The listing builds one solid part. Answer for the finished solid, in the listing's coordinates (mm). A direction names the side the tool comes from. Give positions to 0.01 mm unless a question says otherwise; leave off trailing zeros. Write each loop counter-clockwise with the first axis right and the second up, starting at its lowest first coordinate (ties: lowest second). Pieces come first, ordered by that corner, then holes. Notation, with made-up numbers: (-29.5, 26.5) - (0.5, 26.5) arc R21 cw to (0.5, 57.5) - close; hole circle Ø7 at (81, 60). An arc over 180 degrees is marked (long way). One line per question, with ' | ' between items. Start each with the question number.
1. The mould has two halves that part along X. Classify faces 6 (the face through (0, 0, 0)), 7 (the face through (3.75, 16, 10)), 8 (the face through (-19, 0, 2)), 9 (the face through (20, 0, 12)): +X half, -X half, draft (parallel to the pull), parting line (faces both ways), or undercut.
2. A cutting plane is placed at B-B (z = 16.75). Determine the outline of the cut face in (x, y), then the cut area to 3 significant figures.
3. For faces 1 (the face through (0, -21.5, 10)), 2 (the face through (-3.75, 16, 10)), 3 (the face through (16, 13.9, 11.5)), 4 (the face through (0, 5, 20)), 5 (the face through (-1.19, -16.87, 16.84)), determine the directions among +Z, -Z, +X, -X, +Y, -Y from which every point of the face is accessible in a straight line to the end or side of a thin tool.
4. A cutting plane is placed at C-C (y = 11). Determine the outline of the cut face in (x, z), then the cut area to 3 significant figures.
5. Find the intervals of material crossed by L1, parallel to X at y = 17.5, z = 10; L2, parallel to X at y = 10.75, z = 10; L3, parallel to Z at x = -14, y = 16, in increasing order. Write a range as from..to.
6. Given P1, Ø5.5, axis at x = 0.5, y = -12, coming from the +Z side, flat-ended and moving along its own axis, determine where the tip first touches the part or whether it passes through.
7. A cutting plane is placed at A-A (y = 17.5). Determine the outline of the cut face in (x, z), then the cut area to 3 significant figures.
8. A cutting plane is placed at D-D (z = 11.5). State how many separate pieces and enclosed holes the cut face has, then the cut area to 3 significant figures.
```python
from build123d import *

# Parameters (mm, degrees)
SKETCH1_W                                           = 40
SKETCH1_H                                           = 43
BOSS_EXTRUDE1_DEPTH                                 = 20
SKETCH2_W                                           = 7.5
SKETCH2_H                                           = 20
CUT_EXTRUDE1_DEPTH                                  = 10
M6_TAPPED_HOLE1_D                                   = 5
M6_TAPPED_HOLE1_DEPTH                               = 15
M6_TAPPED_HOLE1_TIP                                 = 1.502151548
FILLET1_R                                           = 5
CHAMFER1_SIZE                                       = 0.5
CBORE_FOR_M6_HEX_SOCKET_HEAD_CAP_SCREW1_D           = 6.4
CBORE_FOR_M6_HEX_SOCKET_HEAD_CAP_SCREW1_CBORE_D     = 11
CBORE_FOR_M6_HEX_SOCKET_HEAD_CAP_SCREW1_CBORE_DEPTH = 6.4
M5_TAPPED_HOLE1_D                                   = 4.2
M5_TAPPED_HOLE1_DEPTH                               = 12.4
M5_TAPPED_HOLE1_TIP                                 = 1.2618073


with BuildPart() as part:
    # Sketch1 → Boss-Extrude1 (new body)
    with BuildSketch(Plane.XY):
        Rectangle(SKETCH1_W, SKETCH1_H)
    extrude(amount=BOSS_EXTRUDE1_DEPTH)

    # Sketch2 → Cut-Extrude1 (cut)
    with BuildSketch(Plane(origin=(0, 21.5, 0), x_dir=(1, 0, 0), z_dir=(0, 1, 0))):
        with Locations((0, -10)):
            Rectangle(SKETCH2_W, SKETCH2_H)
    extrude(amount=-CUT_EXTRUDE1_DEPTH, mode=Mode.SUBTRACT)

    # M6 Tapped Hole1
    with Locations(Plane(origin=(0, 21.5, 0), x_dir=(1, 0, 0), z_dir=(0, 1, 0))):
        with Locations((-14, -10), (14, -10)):
            Hole(M6_TAPPED_HOLE1_D / 2, depth=M6_TAPPED_HOLE1_DEPTH)
            with Locations((0, 0, -(M6_TAPPED_HOLE1_DEPTH + M6_TAPPED_HOLE1_TIP / 2))):  # 118° drill point
                Cone(0, M6_TAPPED_HOLE1_D / 2, M6_TAPPED_HOLE1_TIP, mode=Mode.SUBTRACT)

    # Fillet1
    fillet1_edges = [part.edges().sort_by_distance(p)[0] for p in [
        (-20, 0, 0),
        (20, 0, 0),
    ]]
    fillet(fillet1_edges, radius=FILLET1_R)

    # Chamfer1
    chamfer1_edges = [part.edges().sort_by_distance(p)[0] for p in [
        (-20, 0, 20),
        (-9.375, 21.5, 0),
        (0, -21.5, 20),
        (-11.875, 21.5, 20),
        (-3.75, 21.5, 10),
        (3.75, 21.5, 10),
        (0, -21.5, 0),
        (18.535533906, -21.5, 1.464466094),
        (-18.535533906, -21.5, 1.464466094),
        (9.375, 21.5, 0),
        (-18.535533906, 21.5, 1.464466094),
        (20, 0, 20),
        (18.535533906, 21.5, 1.464466094),
        (20, -21.5, 12.5),
        (-20, -21.5, 12.5),
        (-20, 21.5, 12.5),
        (20, 21.5, 12.5),
        (11.875, 21.5, 20),
    ]]
    chamfer(chamfer1_edges, length=CHAMFER1_SIZE)

    # CBORE for M6 Hex Socket Head Cap Screw1 (through all)
    with Locations(Plane.XY.offset(20)):
        with Locations((0, -11.5)):
            CounterBoreHole(CBORE_FOR_M6_HEX_SOCKET_HEAD_CAP_SCREW1_D / 2, CBORE_FOR_M6_HEX_SOCKET_HEAD_CAP_SCREW1_CBORE_D / 2, CBORE_FOR_M6_HEX_SOCKET_HEAD_CAP_SCREW1_CBORE_DEPTH)

    # M5 Tapped Hole1
    with Locations(Plane.XY.offset(20)):
        with Locations((0, 1.5)):
            Hole(M5_TAPPED_HOLE1_D / 2, depth=M5_TAPPED_HOLE1_DEPTH)
            with Locations((0, 0, -(M5_TAPPED_HOLE1_DEPTH + M5_TAPPED_HOLE1_TIP / 2))):  # 118° drill point
                Cone(0, M5_TAPPED_HOLE1_D / 2, M5_TAPPED_HOLE1_TIP, mode=Mode.SUBTRACT)


solid = part.part
```
Determined:
1) face 6: draft | face 7: undercut | face 8: -X half | face 9: +X half
2) outline: (-20, -21) - (-19.5, -21.5) - (19.5, -21.5) - (20, -21) - (20, 21) - (19.5, 21.5) - (4.25, 21.5) - (3.75, 21) - (3.75, 11.5) - (-3.75, 11.5) - (-3.75, 21) - (-4.25, 21.5) - (-19.5, 21.5) - (-20, 21) - close; hole circle Ø11 at (0, -11.5); hole circle Ø4.2 at (0, 1.5) | area: 1,540 mm2
3) face 1: +Z, -Z, +X, -X, -Y | face 2: +Z, -Z, +Y | face 3: +Y | face 4: +Z, +X, -X, +Y, -Y | face 5: +Z
4) outline: (-20, 5) arc R5 ccw to (-15, 0) - (15, 0) arc R5 ccw to (20, 5) - (20, 19.5) - (19.5, 20) - (-19.5, 20) - (-20, 19.5) - close; hole circle Ø5 at (-14, 10); hole circle Ø5 at (14, 10) | area: 750 mm2
5) L1: -20..-16.5, -11.5..-3.75, 3.75..11.5, 16.5..20 | L2: -20..-16.5, -11.5..11.5, 16.5..20 | L3: 0..7.5, 12.5..20
6) P1: z = 13.6
7) outline: (-20, 5) arc R5 ccw to (-15, 0) - (-3.75, 0) - (-3.75, 20) - (-19.5, 20) - (-20, 19.5) - close; (3.75, 0) - (15, 0) arc R5 ccw to (20, 5) - (20, 19.5) - (19.5, 20) - (3.75, 20) - close; hole circle Ø5 at (-14, 10); hole circle Ø5 at (14, 10) | area: 600 mm2
8) separate pieces: 1 | enclosed holes: 2 | area: 1,480 mm2
